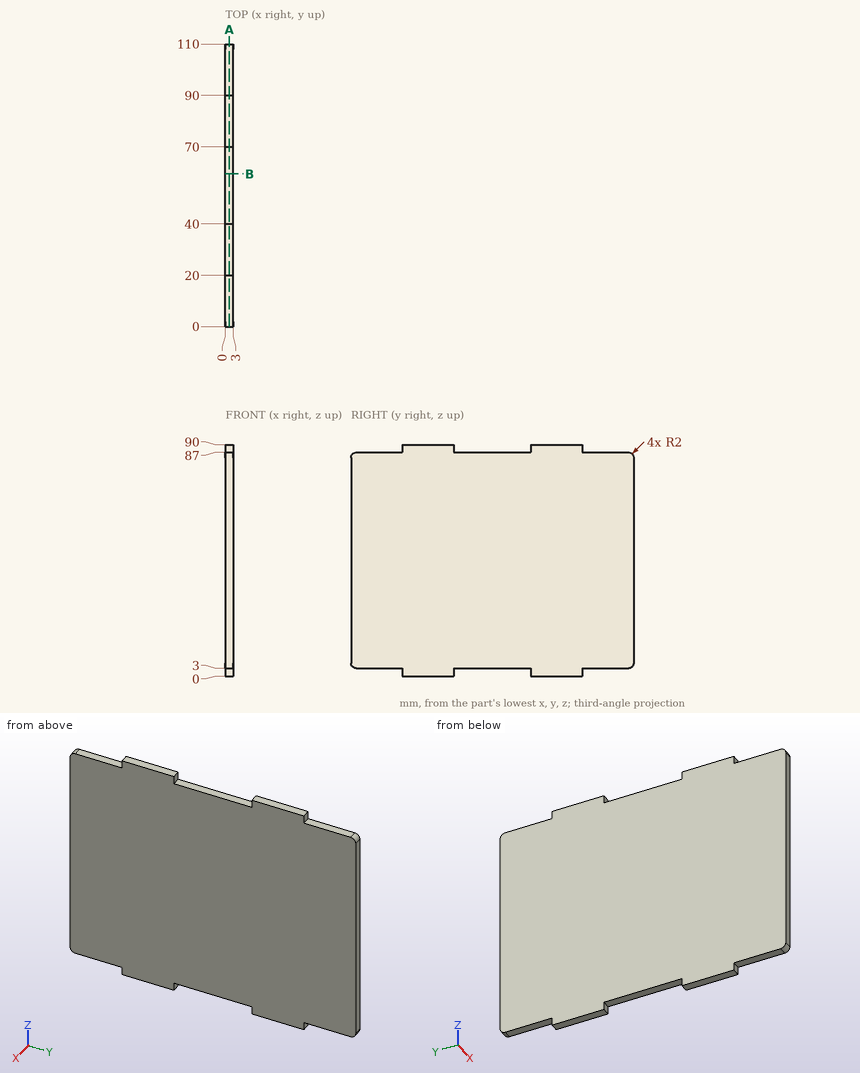
Job drawing, mm, ordinate dimensions from the low corner. One solid piece. Round coordinates to 2 decimals unless told otherwise and drop trailing zeros. Loops run counter-clockwise (first coordinate to the right, second up) from the corner with the lowest first, then second, coordinate; pieces in that order, holes last. Notation, with made-up numbers: (-17.75, 11.25) -> (-12.75, 11.25) arc R6 ccw to (-12.75, 19.25) -> close; hole circle Ø9 at (-39, 42). An arc over 180 degrees is marked (long way). Use a Markdown table: item, result.
1) Cut at B-B, the plane y = 59.5. List the corners of the cut face in (x, z).
The answers:
| item | result |
|---|---|
| outline | (0, 3) -> (3, 3) -> (3, 87) -> (0, 87) -> close |
2) Drop flat-ended pins along their axis: pin 1 Ø0.9 at (x, y) = (1, 101) entering from +Z; pin 2 Ø1.5 at (x, z) = (2, 89) entering from +Y; pin 3 Ø0.9 at (x, y) = (1.5, 94.5) entering from -Z. Give the stop position or say it passes through.
The answers:
| item | result |
|---|---|
| pin 1 | stops at z = 87 |
| pin 2 | stops at y = 90 |
| pin 3 | stops at z = 3 |
3) Cut at A-A, the plane x = 1.6. List the corners of the cut face in (y, z).
The answers:
| item | result |
|---|---|
| outline | (0, 5) arc R2 ccw to (2, 3) -> (20, 3) -> (20, 0) -> (40, 0) -> (40, 3) -> (70, 3) -> (70, 0) -> (90, 0) -> (90, 3) -> (108, 3) arc R2 ccw to (110, 5) -> (110, 85) arc R2 ccw to (108, 87) -> (90, 87) -> (90, 90) -> (70, 90) -> (70, 87) -> (40, 87) -> (40, 90) -> (20, 90) -> (20, 87) -> (2, 87) arc R2 ccw to (0, 85) -> close |
4) Probe line 1 (Z direction, x = 1.5, y = 9); line 2 (Y direction, x = 2.8, z = 4.5). List the from-to ranges inside material, lowest first. Write a range as [from, to].
The answers:
| item | result |
|---|---|
| line 1 | z = [3, 87] |
| line 2 | y = [0.06, 109.94] |
